Part print with two shaded views. Sizes in mm from the minimum x, y, z corner. Coordinates: 2 decimals unless noted, no trailing zeros. Order: outer loops, then holes, each group sorted by start corner. A loop starts at its lowest first (then second) coordinate and runs counter-clockwise, first axis right, second up.
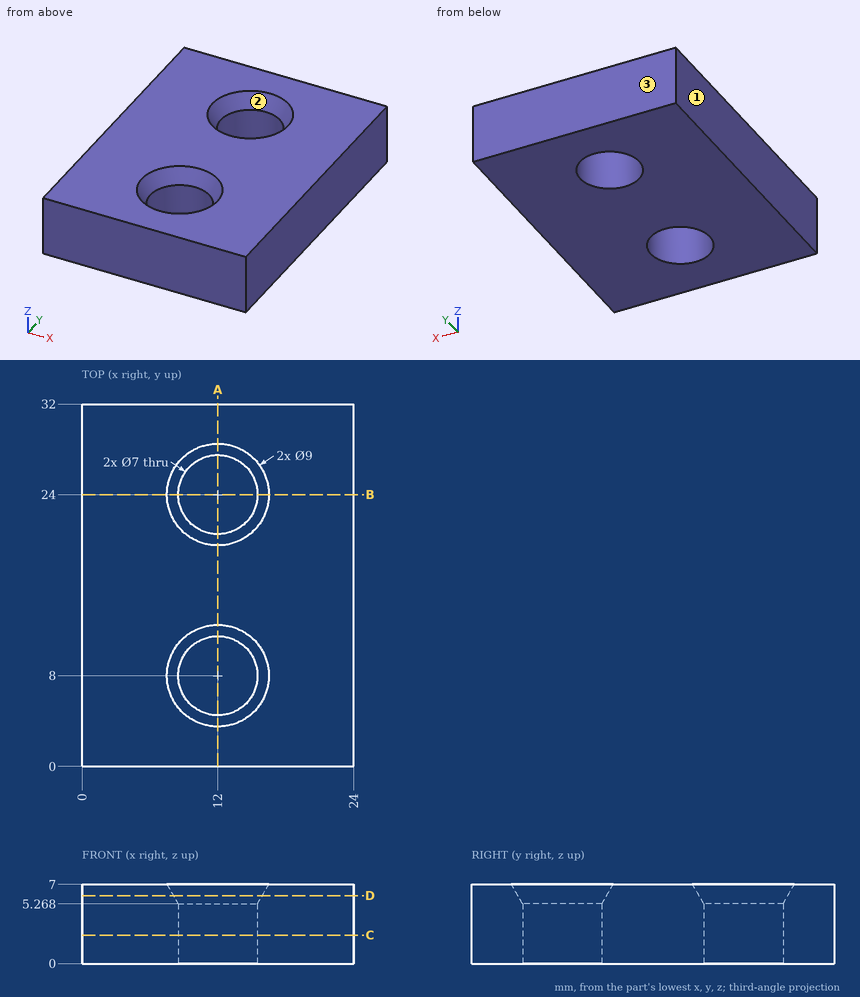
Q1. Cut at D-D on z = 6. Write the cut outline in (x, y).
Results list:
outline: (0, 0) - (24, 0) - (24, 32) - (0, 32) - close; hole circle Ø7.85 at (12, 8); hole circle Ø7.85 at (12, 24)
Q2. Wall check: line 1 along Y through (x, z) = (12, 3.8); line 2 along X through (y, z) = (24, 1.85); line 3 along Y through (x, z) = (9.75, 5.75). Give the ranges that are in metal, low to high.
Results list:
line 1: y = 0 to 4.5, 11.5 to 20.5, 27.5 to 32
line 2: x = 0 to 8.5, 15.5 to 24
line 3: y = 0 to 4.96, 11.04 to 20.96, 27.04 to 32
Q3. Mould opens along X. For the marked faces 1, 2 and 3 say: pulls with the +X half, pulls with the -X half, needs draft (parallel to the pull), parting line crosses it, or undercut.
Results list:
face 1: pulls with the -X half
face 2: undercut
face 3: needs draft
Q4. Cut at C-C on z = 2.5. Write the cut outline in (x, y), and give its area (3 significant figures).
Results list:
outline: (0, 0) - (24, 0) - (24, 32) - (0, 32) - close; hole circle Ø7 at (12, 8); hole circle Ø7 at (12, 24)
area: 691 mm2
Q5. Cut at B-B on y = 24. Write the cut outline in (x, z), and give its area (3 significant figures).
Results list:
outline: (0, 0) - (8.5, 0) - (8.5, 5.27) - (7.5, 7) - (0, 7) - close; (15.5, 0) - (24, 0) - (24, 7) - (16.5, 7) - (15.5, 5.27) - close
area: 117 mm2
Q6. Cut at A-A on x = 12. Write the cut outline in (y, z), and give its area (3 significant figures).
Results list:
outline: (0, 0) - (4.5, 0) - (4.5, 5.27) - (3.5, 7) - (0, 7) - close; (11.5, 0) - (20.5, 0) - (20.5, 5.27) - (19.5, 7) - (12.5, 7) - (11.5, 5.27) - close; (27.5, 0) - (32, 0) - (32, 7) - (28.5, 7) - (27.5, 5.27) - close
area: 123 mm2
